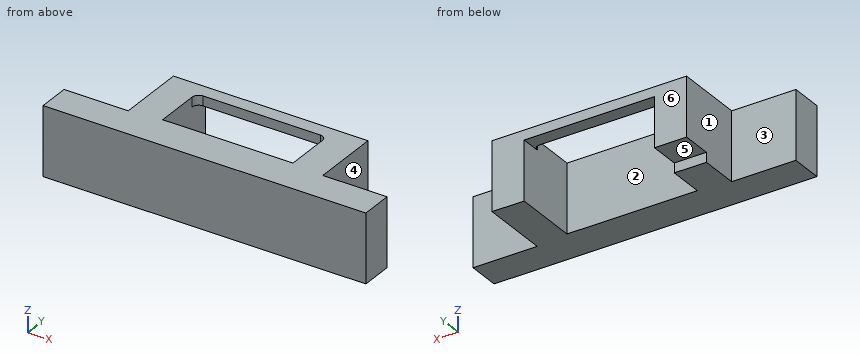
from build123d import *

# Parameters (mm, degrees)
CROQUIS1_W              = 50.3
CROQUIS1_H              = 10.7
SALIENTE_EXTRUIR1_DEPTH = 15.7
CORTAR_EXTRUIR1_REACH   = 55.769
CROQUIS2_W              = 10
CROQUIS2_H              = 10.7
CORTAR_EXTRUIR2_REACH   = 55.769
CROQUIS3_W              = 20.3
CROQUIS3_H              = 9.2
CORTAR_EXTRUIR3_REACH   = 46.554
CROQUIS4_W              = 1.5
CROQUIS4_H              = 4.7


with BuildPart() as part:
    # Croquis1 → Saliente-Extruir1 (new body)
    with BuildSketch(Plane(origin=(0, 0, 0), x_dir=(1, 0, 0), z_dir=(0, 1, 0))):
        with Locations((-25.15, -5.35)):
            Rectangle(CROQUIS1_W, CROQUIS1_H)
    extrude(amount=SALIENTE_EXTRUIR1_DEPTH)

    # Croquis2 → Cortar-Extruir1 (cut, up to next)
    with BuildSketch(Plane.XY.offset(10.7), mode=Mode.PRIVATE) as cortar_extruir1_sk1:
        with Locations((-45.3, 10.35)):
            Rectangle(CROQUIS2_W, CROQUIS2_H)
    cortar_extruir1_tool1 = extrude(cortar_extruir1_sk1.sketch, amount=-CORTAR_EXTRUIR1_REACH, mode=Mode.PRIVATE) & part.part
    # Croquis2 → Cortar-Extruir1 (cut, up to next)
    with BuildSketch(Plane.XY.offset(10.7), mode=Mode.PRIVATE) as cortar_extruir1_sk2:
        with BuildLine():
            Line((-35.3, 5.532906309), (-15, 5.532906309))
            Line((-15, 5.532906309), (-15, 12.532906309))
            ThreePointArc((-15, 12.532906309), (-15.292893219, 13.240013091), (-16, 13.532906309))
            Line((-16, 13.532906309), (-34.3, 13.532906309))
            ThreePointArc((-34.3, 13.532906309), (-35.007106781, 13.240013091), (-35.3, 12.532906309))
            Line((-35.3, 12.532906309), (-35.3, 5.532906309))
        make_face()
    cortar_extruir1_tool2 = extrude(cortar_extruir1_sk2.sketch, amount=-CORTAR_EXTRUIR1_REACH, mode=Mode.PRIVATE) & part.part
    # Croquis2 → Cortar-Extruir1 (cut, up to next)
    with BuildSketch(Plane.XY.offset(10.7), mode=Mode.PRIVATE) as cortar_extruir1_sk3:
        with Locations((-5, 10.35)):
            Rectangle(CROQUIS2_W, CROQUIS2_H)
    cortar_extruir1_tool3 = extrude(cortar_extruir1_sk3.sketch, amount=-CORTAR_EXTRUIR1_REACH, mode=Mode.PRIVATE) & part.part
    add(cortar_extruir1_tool1.solids().sort_by_distance((-45.3, 10.35, 10.7))[0], mode=Mode.SUBTRACT)
    add(cortar_extruir1_tool2.solids().sort_by_distance((-25.15, 9.522899, 10.7))[0], mode=Mode.SUBTRACT)
    add(cortar_extruir1_tool3.solids().sort_by_distance((-5, 10.35, 10.7))[0], mode=Mode.SUBTRACT)

    # Croquis3 → Cortar-Extruir2 (cut, up to next)
    with BuildSketch(Plane(origin=(0, 15.7, 0), x_dir=(1, 0, 0), z_dir=(0, 1, 0)), mode=Mode.PRIVATE) as cortar_extruir2_sk1:
        with Locations((-25.15, -4.6)):
            Rectangle(CROQUIS3_W, CROQUIS3_H)
    cortar_extruir2_tool1 = extrude(cortar_extruir2_sk1.sketch, amount=-CORTAR_EXTRUIR2_REACH, mode=Mode.PRIVATE) & part.part
    add(cortar_extruir2_tool1.solids().sort_by_distance((-25.15, 15.7, 4.6))[0], mode=Mode.SUBTRACT)

    # Croquis4 → Cortar-Extruir3 (cut, up to next)
    with BuildSketch(Plane.ZY.offset(40.3), mode=Mode.PRIVATE) as cortar_extruir3_sk1:
        with Locations((0.75, 13.35)):
            Rectangle(CROQUIS4_W, CROQUIS4_H)
    cortar_extruir3_tool1 = extrude(cortar_extruir3_sk1.sketch, amount=-CORTAR_EXTRUIR3_REACH, mode=Mode.PRIVATE) & part.part
    add(cortar_extruir3_tool1.solids().sort_by_distance((-40.3, 13.35, 0.75))[0], mode=Mode.SUBTRACT)


solid = part.part
Geometry check sheet. Reference: the model listing, model coordinates, mm. Face numbers are marked on the shaded views. A direction names the side the tool comes from. Round coordinates to 2 decimals unless told otherwise and drop trailing zeros. Write each loop counter-clockwise with the first axis right and the second up, starting at its lowest first coordinate (ties: lowest second). Pieces come first, ordered by that corner, then holes. Notation, with made-up numbers: (81, 44) - (138, 44) arc R25 cw to (138, 63) - close; hole circle Ø6 at (18.25, 76.5). An arc over 180 degrees is marked (long way). One line per item, written item: value.
1. Cross-section at B-B on y = 9. Record the boundary of the cut face in (x, z).
The answers:
outline: (-40.3, 0) - (-35.3, 0) - (-35.3, 10.7) - (-40.3, 10.7) - close; (-15, 0) - (-10, 0) - (-10, 10.7) - (-15, 10.7) - close
2. Cross-section at C-C on z = 4.75. Record the boundary of the cut face in (x, y).
The answers:
outline: (-50.3, 0) - (0, 0) - (0, 5) - (-10, 5) - (-10, 15.7) - (-15, 15.7) - (-15, 5.53) - (-35.3, 5.53) - (-35.3, 15.7) - (-40.3, 15.7) - (-40.3, 5) - (-50.3, 5) - close
3. Set-up check for the marked faces 4, 5 and 6: record each of +Z, -Z, +X, -X, +Y, -Y from which the full face is reachable in a straight line by a thin tool's end or side.
The answers:
face 4: +Z, -Z, +X, +Y
face 5: -Z, -X, +Y
face 6: +Z, -Z, +X, -X, +Y
4. Cross-section at A-A on x = -33. Record the boundary of the cut face in (y, z).
The answers:
outline: (0, 0) - (5.53, 0) - (5.53, 10.7) - (0, 10.7) - close; (13.53, 9.2) - (15.7, 9.2) - (15.7, 10.7) - (13.53, 10.7) - close
5. Depth check by flat-ended pin: pin 1 Ø3 at (x, z) = (-25, 3) entering from +Y; pin 2 Ø3 at (y, z) = (10, 3) entering from -X; pin 3 Ø0.8 at (x, z) = (-38.5, 0.5) entering from +Y. Enter the tip coordinate at first touch or a pass-through.
The answers:
pin 1: stops at y = 5.53
pin 2: stops at x = -40.3
pin 3: stops at y = 11
6. Cross-section at D-D on y = 14. Record the boundary of the cut face in (x, z), and give its area (3 significant figures).
The answers:
outline: (-40.3, 1.5) - (-35.3, 1.5) - (-35.3, 9.2) - (-15, 9.2) - (-15, 0) - (-10, 0) - (-10, 10.7) - (-40.3, 10.7) - close
area: 130 mm^2
7. Scan lines: L1, parallel to X at y = 11.25, z = 3.5; L2, parallel to Y at x = -21.5, z = 10; L3, parallel to Y at x = -47, z = 6.5. Record each from-to range of solid material in increasing order.
The answers:
L1: x = -40.3 to -35.3, -15 to -10
L2: y = 0 to 5.53, 13.53 to 15.7
L3: y = 0 to 5
8. Mould release check, pull along X, two halves, no side actions. Record for the marked faces 1, 2 and 3: released by +X, released by -X, zero draft, split by the parting line, or undercut.
The answers:
face 1: released by -X
face 2: undercut
face 3: zero draft
